Verification items for the finished model (mm, model axes). Face numbers are marked on the shaded views. A direction names the side the tool comes from. Round coordinates to 2 decimals unless told otherwise and drop trailing zeros. Write each loop counter-clockwise with the first axis right and the second up, starting at its lowest first coordinate (ties: lowest second). Pieces come first, ordered by that corner, then holes. Notation, with made-up numbers: M 31,23.5 L 58,23.5 A15 ccw 58,50.5 Z; hole C 29,28.5 d8. An arc over 180 degrees is marked long. One line per item, written item: value. Start each with the question number.
from build123d import *

# Parameters (mm, degrees)
F0_R          = 3
F0_R_2        = 1.75
F1_DEPTH      = 16
F1_DEPTH_BACK = 2.99974
F2_R          = 1.75
F3_DEPTH      = 3
F5_DEPTH      = 6
F7_DEPTH      = 50
F10_DEPTH     = 6
F8_R          = 1.75
F11_DEPTH     = 72.00074
F12_R         = 1.75
F13_DEPTH     = 2.99974
F14_W         = 3
F14_H         = 3
F15_DEPTH     = 24
F17_DEPTH     = 3
F18_R         = 10
F18_R_2       = 7
F19_DEPTH     = 3
F21_DEPTH     = 3
F22_R         = 7
F23_DEPTH     = 25.4


with BuildPart() as f1:
    # F0 (on Front) → F1 (new body, two sides)
    with BuildSketch(Plane.XZ) as f1_sk:
        Circle(F0_R)
        Circle(F0_R_2, mode=Mode.SUBTRACT)
    extrude(amount=F1_DEPTH)
    extrude(f1_sk.sketch, amount=-F1_DEPTH_BACK)

    # F2 (on face) → F3 (join)
    with BuildSketch(Plane.XZ.offset(16)):
        with BuildLine():
            Line((-3, 30), (-3, 0))
            ThreePointArc((-3, 0), (0, -3), (3, 0))
            Line((3, 0), (3, 30))
            ThreePointArc((3, 30), (0, 33), (-3, 30))
        make_face()
        with Locations((0, 30)):
            Circle(F2_R, mode=Mode.SUBTRACT)
    extrude(amount=F3_DEPTH)

    # F4 (on face) → F5 (join, through all)
    with BuildSketch(Plane(origin=(-3, 0, 0), x_dir=(0, -1, 0), z_dir=(-1, 0, 0))):
        Polygon((69, 0), (19, 27), (19, 0), align=None)
    extrude(amount=-F5_DEPTH)

    # F6 (on face) → F7 (join, through all)
    with BuildSketch(Plane.XZ.offset(19)):
        with BuildLine():
            Line((3, 0), (-3, 0))
            ThreePointArc((-3, 0), (0, -3), (3, 0))
        make_face()
    extrude(amount=F7_DEPTH)

    # F9 (on face) → F10 (join)
    with BuildSketch(Plane.XZ.offset(69)):
        with BuildLine():
            Line((-3, 3.128744429), (-3, 0))
            ThreePointArc((-3, 0), (0, -3), (3, 0))
            Line((3, 0), (3, 3.128744429))
            Line((3, 3.128744429), (-3, 3.128744429))
        make_face()
    extrude(amount=-F10_DEPTH)

    # F8 (on face) → F11 (cut, through all)
    with BuildSketch(Plane(origin=(0, 2.99974, 0), x_dir=(-1, 0, 0), z_dir=(0, 1, 0))):
        Circle(F8_R)
    extrude(amount=-F11_DEPTH, mode=Mode.SUBTRACT)



with BuildPart() as f13:
    # F12 (on face) → F13 (new body)
    with BuildSketch(Plane.XZ.offset(19)):
        with BuildLine():
            Line((33, 27), (33, 30))
            ThreePointArc((33, 30), (30, 33), (27, 30))
            Line((27, 30), (27, 27))
            Line((27, 27), (33, 27))
        make_face()
        with Locations((30, 30)):
            Circle(F12_R, mode=Mode.SUBTRACT)
    extrude(amount=-F13_DEPTH)


with BuildPart() as f1_1:
    add(f1.part)

    add(f13.part)  # F15 merges F13
    # F14 (on face) → F15 (join, through all)
    with BuildSketch(Plane.YZ.offset(3)):
        with Locations((-17.5, 28.5)):
            Rectangle(F14_W, F14_H)
    extrude(amount=F15_DEPTH)

    # F16 (on face) → F17 (join, through all)
    with BuildSketch(Plane(origin=(0, -16, 0), x_dir=(-1, 0, 0), z_dir=(0, 1, 0))):
        Polygon((-27, 27), (-33, 27), (-3, 0), (-3, 5.4), align=None)
    extrude(amount=-F17_DEPTH)

    # F18 (on face) → F19 (join, through all)
    with BuildSketch(Plane(origin=(0, -16, 0), x_dir=(-1, 0, 0), z_dir=(0, 1, 0))):
        with Locations((-16.5, 14.85)):
            Circle(F18_R)
        with Locations((-16.5, 14.85)):
            Circle(F18_R_2, mode=Mode.SUBTRACT)
    extrude(amount=-F19_DEPTH)

    # F20 (on face) → F21 (join, through all)
    with BuildSketch(Plane(origin=(0, -16, 0), x_dir=(-1, 0, 0), z_dir=(0, 1, 0))):
        with BuildLine():
            Line((-8.5159330462, 20.8711855043), (-3, 27))
            Line((-3, 27), (-8.99948, 27))
            Line((-8.99948, 27), (-11.9295075041, 23.7444138843))
            ThreePointArc((-11.9295075041, 23.7444138843), (-10.0604269493, 22.5006142842), (-8.5159330462, 20.8711855043))
        make_face()
    extrude(amount=-F21_DEPTH)

    # F22 (on face) → F23 (cut)
    with BuildSketch(Plane(origin=(0, -16, 0), x_dir=(-1, 0, 0), z_dir=(0, 1, 0))):
        with Locations((-16.5, 14.85)):
            Circle(F22_R)
    extrude(amount=-F23_DEPTH, mode=Mode.SUBTRACT)


solid = f1_1.part
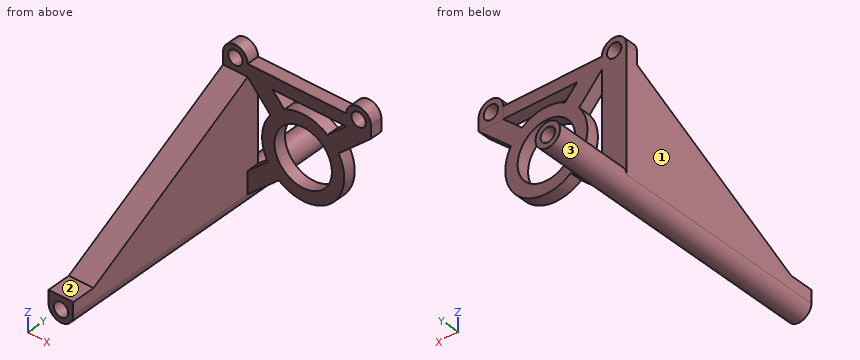
1) Gauge pin test, flat ends, axial feed: pin 1 Ø1.7 at (x, y) = (0.5, -65) entering from +Z; pin 2 Ø4 at (x, z) = (1, 23) entering from +Y; pin 3 Ø2.5 at (x, y) = (9, -18) entering from +Z; pin 4 Ø4.5 at (x, z) = (0, 0) entering from -Y. Record the tip position at first contact, or that the pin passes through.
2) Access from +Z, -Z, +X, -X, +Y, -Y to the whole of each face (thin tool, end or side, straight path). Record for the marked faces 1, 2 and 3.
3) Thickness scan on line 1 (Z direction, x = 0, y = -17.05); line 2 (Z direction, x = 16.5, y = -17.85); line 3 (X direction, y = -17.5, z = 14.5). Record the ranges inside material, lowest first.
4) Cross-section at A-A (x = 16.5). Record the boundary of the cut face in (y, z).
5) Cross-section at B-B (z = 14.85). Record the boundary of the cut face in (x, y), then the cut area to 3 significant figures.
6) Cross-section at D-D (y = -39.5). Record the boundary of the cut face in (x, z), then the cut area to 3 significant figures.
Results below:
1. pin 1: stops at z = 3.13
1. pin 2: stops at y = -16
1. pin 3: stops at z = 30
1. pin 4: stops at y = -69
2. face 1: +Z, -Z, -X, +Y, -Y
2. face 2: +Z, +X, -X, -Y
2. face 3: +Y
3. line 1: z = -3 to -1.75, 1.75 to 28.25, 31.75 to 33
3. line 2: z = 4.85 to 7.85, 21.85 to 24.85, 27 to 30
3. line 3: x = -3 to 3, 6.51 to 9.51, 23.49 to 26.49
4. outline: M -19,4.85 L -16,4.85 L -16,7.85 L -19,7.85 Z; M -19,21.85 L -16,21.85 L -16,24.85 L -19,24.85 Z; M -19,27 L -16,27 L -16,30 L -19,30 Z
5. outline: M -3,-41.5 L 3,-41.5 L 3,-16 L -3,-16 Z; M 6.5,-19 L 9.5,-19 L 9.5,-16 L 6.5,-16 Z; M 23.5,-19 L 26.5,-19 L 26.5,-16 L 23.5,-16 Z
5. area: 171 mm²
6. outline: M -3,0 A3 ccw 3,0 L 3,15.93 L -3,15.93 Z; hole C 0,0 d3.5
6. area: 100 mm²
